Part model, mm, in its own coordinate system. A direction names the side the tool comes from. Coordinates: 2 decimals unless noted, no trailing zeros. Loops run counter-clockwise (first coordinate to the right, second up) from the corner with the lowest first, then second, coordinate; pieces in that order, holes last. Notation, with made-up numbers: (58.5, 59.25) -> (102.5, 59.25) arc R29 cw to (102.5, 82.25) -> close; hole circle Ø1 at (-36, -18.75). An arc over 180 degrees is marked (long way). Use one line per item in the form item = value. Start each with the question number.
(1) Mould opens along Z. For faces 1 (the flat face through (0, 39, 2)), 2 (the cylindrical face through (-37.1, -37.14, 3.45)), 3 (the flat face through (-1, 1, 10)) say: +Z half, -Z half, draft (parallel to the pull), parting line (faces both ways), or undercut.
(2) Band-saw the part on C-C on y = 7.5. Give the cut face in (x, z).
(3) Pin check, flat tips, straight feed: P1, Ø1.6, axis at x = -38.5, z = 6, coming from the -Y side; P2, Ø1.8, axis at x = -20, y = -25.5, coming from the -Z side; P3, Ø1, axis at x = -7, y = 9, coming from the -Z side. Stop position of each tip, or through.
(4) 3-axis set-ups, long thin cutter, end or side, ignore diameter. For faces 4 (the flat face through (-39, -8, 3)), 5 (the flat face through (-10, -39, 6)), 6 (the cylindrical face through (-21.445, -27.737, 2.014)), 7 (the cylindrical face through (-37.14, 37.1, 4.23)), 8 (the flat face through (-22, -39, 5)): which of +Z, -Z, +X, -X, +Y, -Y reach the whole face in a straight line?
(5) Drill centre lines: L1, parallel to X at y = 0, z = 4.9; L2, parallel to Y at x = -18, z = 4.2; L3, parallel to Y at x = -18, z = 5.85. Where is each one in solid material? Low to high. Write a range as [from, to].
(6) Band-saw the part on A-A on y = -14. Give the cut face in (x, z).
(7) Band-saw the part on D-D on y = 26.25. Give the cut face in (x, z), then the cut area to 3 significant figures.
```python
from build123d import *

# Parameters (mm, degrees)
PAD_DEPTH       = 10
FILLET_R        = 2.5
SKETCH002_W     = 20
SKETCH002_H     = 2
POCKET_DEPTH    = 2
POCKET001_DEPTH = 7
SKETCH013_R     = 3
PAD007_DEPTH    = 4
SKETCH014_R     = 1.5
PAD008_DEPTH    = 2
SKETCH015_W     = 25
SKETCH015_H     = 2
POCKET004_DEPTH = 2
SKETCH016_W     = 25
SKETCH016_H     = 2
POCKET005_DEPTH = 2
SKETCH017_W     = 20
SKETCH017_H     = 2
POCKET006_DEPTH = 2
SKETCH018_R     = 1.4
POCKET007_DEPTH = 4
SKETCH023_W     = 5.5
SKETCH023_H     = 1.6
PAD011_DEPTH    = 1.5
CHAMFER001_SIZE = 0.2
SKETCH024_W     = 2.2
SKETCH024_H     = 4.2
POCKET011_DEPTH = 0.5


with BuildPart() as part:
    # Sketch → Pad (new body)
    with BuildSketch(Plane.XY):
        with BuildLine():
            Line((-34.999972, -40), (34.999972, -40))
            ThreePointArc((34.999972, -40), (38.535524, -38.535544), (40, -35))
            Line((40, 35), (40, -35))
            ThreePointArc((40, 35), (38.535534, 38.535534), (35, 40))
            Line((35, 40), (-35, 40))
            ThreePointArc((-35, 40), (-38.535534, 38.535534), (-40, 35))
            Line((-40, 35), (-40, -35))
            ThreePointArc((-40, -35), (-38.535524, -38.535544), (-34.999972, -40))
        make_face()
    extrude(amount=PAD_DEPTH)

    # Fillet
    fillet_edges = [part.edges().sort_by_distance(p)[0] for p in [
        (38.535534, 38.535534, 10),
        (0, 40, 10),
        (-38.535534, 38.535534, 10),
        (-40, 0, 10),
        (-38.535524, -38.535544, 10),
        (0, -40, 10),
        (38.535524, -38.535544, 10),
        (40, 0, 10),
    ]]
    fillet(fillet_edges, radius=FILLET_R)

    # Sketch002 → Pocket (cut)
    with BuildSketch(Plane.XZ.offset(40)):
        with Locations((0, 3)):
            Rectangle(SKETCH002_W, SKETCH002_H)
        with Locations((0, 6)):
            Rectangle(SKETCH002_W, SKETCH002_H)
        with Locations((-22, 3)):
            Rectangle(SKETCH002_W, SKETCH002_H)
        with Locations((-22, 6)):
            Rectangle(SKETCH002_W, SKETCH002_H)
        with Locations((22, 6)):
            Rectangle(SKETCH002_W, SKETCH002_H)
        with Locations((22, 3)):
            Rectangle(SKETCH002_W, SKETCH002_H)
    extrude(amount=-POCKET_DEPTH, mode=Mode.SUBTRACT)

    # Sketch003 → Pocket001 (cut)
    with BuildSketch(Plane(origin=(0, 0, 0), x_dir=(1, 0, 0), z_dir=(0, 0, -1))):
        with BuildLine():
            ThreePointArc((38, 34.999972), (37.121312, 37.121312), (34.999972, 38))
            Line((-35, 38), (34.999972, 38))
            ThreePointArc((-35, 38), (-37.12132, 37.12132), (-38, 35))
            Line((-38, -35.000001), (-38, 35))
            ThreePointArc((-38, -35.000001), (-37.12132, -37.121321), (-35, -38))
            Line((34.999987, -38), (-35, -38))
            ThreePointArc((34.999987, -38), (37.121316, -37.121316), (38, -34.999986))
            Line((38, 34.999972), (38, -34.999986))
        make_face()
    extrude(amount=-POCKET001_DEPTH, mode=Mode.SUBTRACT)

    # Sketch013 → Pad007 (new body)
    with BuildSketch(Plane(origin=(0, 0, 7), x_dir=(1, 0, 0), z_dir=(0, 0, -1))):
        with Locations((-21.25, 26.25)):
            Circle(SKETCH013_R)
        with Locations((21.25, 26.25)):
            Circle(SKETCH013_R)
        with Locations((-21.25, -26.25)):
            Circle(SKETCH013_R)
        with Locations((21.25, -26.25)):
            Circle(SKETCH013_R)
        with Locations((-18, 0)):
            Circle(SKETCH013_R)
        with Locations((18, 0)):
            Circle(SKETCH013_R)
    extrude(amount=PAD007_DEPTH)

    # Sketch014 → Pad008 (new body)
    with BuildSketch(Plane(origin=(0, 0, 3), x_dir=(1, 0, 0), z_dir=(0, 0, -1))):
        with Locations((-21.25, 26.25)):
            Circle(SKETCH014_R)
        with Locations((21.25, 26.25)):
            Circle(SKETCH014_R)
        with Locations((-21.25, -26.25)):
            Circle(SKETCH014_R)
        with Locations((21.25, -26.25)):
            Circle(SKETCH014_R)
    extrude(amount=PAD008_DEPTH)

    # Sketch015 → Pocket004 (cut)
    with BuildSketch(Plane(origin=(-40, 0, 0), x_dir=(0, -1, 0), z_dir=(-1, 0, 0))):
        with Locations((20.5, 3)):
            Rectangle(SKETCH015_W, SKETCH015_H)
        with Locations((20.5, 6)):
            Rectangle(SKETCH015_W, SKETCH015_H)
    extrude(amount=-POCKET004_DEPTH, mode=Mode.SUBTRACT)

    # Sketch016 → Pocket005 (cut)
    with BuildSketch(Plane.YZ.offset(40)):
        with Locations((-20.5, 3)):
            Rectangle(SKETCH016_W, SKETCH016_H)
        with Locations((-20.5, 6)):
            Rectangle(SKETCH016_W, SKETCH016_H)
    extrude(amount=-POCKET005_DEPTH, mode=Mode.SUBTRACT)

    # Sketch017 → Pocket006 (cut)
    with BuildSketch(Plane(origin=(0, 40, 0), x_dir=(-1, 0, 0), z_dir=(0, 1, 0))):
        with Locations((0, 3)):
            Rectangle(SKETCH017_W, SKETCH017_H)
        with Locations((0, 6)):
            Rectangle(SKETCH017_W, SKETCH017_H)
        with Locations((-22, 3)):
            Rectangle(SKETCH017_W, SKETCH017_H)
        with Locations((-22, 6)):
            Rectangle(SKETCH017_W, SKETCH017_H)
        with Locations((22, 6)):
            Rectangle(SKETCH017_W, SKETCH017_H)
        with Locations((22, 3)):
            Rectangle(SKETCH017_W, SKETCH017_H)
    extrude(amount=-POCKET006_DEPTH, mode=Mode.SUBTRACT)

    # Sketch018 → Pocket007 (cut)
    with BuildSketch(Plane(origin=(0, 0, 3), x_dir=(1, 0, 0), z_dir=(0, 0, -1))):
        with Locations((-18, 0)):
            Circle(SKETCH018_R)
        with Locations((18, 0)):
            Circle(SKETCH018_R)
    extrude(amount=-POCKET007_DEPTH, mode=Mode.SUBTRACT)

    # Sketch023 → Pad011 (new body)
    with BuildSketch(Plane.XZ.offset(-38)):
        with Locations((34.749987, 3)):
            Rectangle(SKETCH023_W, SKETCH023_H)
        with Locations((-34.75, 3)):
            Rectangle(SKETCH023_W, SKETCH023_H)
    extrude(amount=PAD011_DEPTH)

    # Chamfer001
    chamfer001_edges = [part.edges().sort_by_distance(p)[0] for p in [
        (34.749987, 36.5, 2.2),
        (-34.75, 36.5, 3.8),
        (-34.75, 36.5, 2.2),
        (34.749987, 36.5, 3.8),
    ]]
    chamfer(chamfer001_edges, length=CHAMFER001_SIZE)

    # Sketch024 → Pocket011 (cut)
    with BuildSketch(Plane(origin=(0, -38, 0), x_dir=(-1, 0, 0), z_dir=(0, 1, 0))):
        with Locations((-33.999972, 3)):
            Rectangle(SKETCH024_W, SKETCH024_H)
        with Locations((34, 3)):
            Rectangle(SKETCH024_W, SKETCH024_H)
    extrude(amount=-POCKET011_DEPTH, mode=Mode.SUBTRACT)


solid = part.part
```
A:
q1.face_1 = undercut
q1.face_2 = draft
q1.face_3 = +Z half
q2.outline = (-40, 0) -> (-38, 0) -> (-38, 7) -> (38, 7) -> (38, 0) -> (40, 0) -> (40, 7.5) arc R2.5 ccw to (37.5, 10) -> (-37.5, 10) arc R2.5 ccw to (-40, 7.5) -> close
q3.P1 = -39.21
q3.P2 = 1
q3.P3 = 7
q4.face_4 = +X, -X
q4.face_5 = +Y, -Y
q4.face_6 = -Z
q4.face_7 = none
q4.face_8 = -Y
q5.L1 = [-40, -38], [-21, -19.4], [-16.6, -15], [15, 16.6], [19.4, 21], [38, 40]
q5.L2 = [-40, -38], [-3, -1.4], [1.4, 3], [38, 40]
q5.L3 = [-3, -1.4], [1.4, 3]
q6.outline = (-40, 0) -> (-38, 0) -> (-38, 2) -> (-40, 2) -> close; (-40, 4) -> (-38, 4) -> (-38, 5) -> (-40, 5) -> close; (-40, 7) -> (40, 7) -> (40, 7.5) arc R2.5 ccw to (37.5, 10) -> (-37.5, 10) arc R2.5 ccw to (-40, 7.5) -> close; (38, 0) -> (40, 0) -> (40, 2) -> (38, 2) -> close; (38, 4) -> (40, 4) -> (40, 5) -> (38, 5) -> close
q7.outline = (-40, 0) -> (-38, 0) -> (-38, 7) -> (-24.25, 7) -> (-24.25, 3) -> (-22.75, 3) -> (-22.75, 1) -> (-19.75, 1) -> (-19.75, 3) -> (-18.25, 3) -> (-18.25, 7) -> (18.25, 7) -> (18.25, 3) -> (19.75, 3) -> (19.75, 1) -> (22.75, 1) -> (22.75, 3) -> (24.25, 3) -> (24.25, 7) -> (38, 7) -> (38, 0) -> (40, 0) -> (40, 7.5) arc R2.5 ccw to (37.5, 10) -> (-37.5, 10) arc R2.5 ccw to (-40, 7.5) -> close
q7.area = 325 mm²
